```python
from build123d import *

# Parameters (mm, degrees)
MAIN_PROFILE_SKETCH_R    = 1.7
MAIN_EXTRUSION_DEPTH     = 4
DETAIL_EXTRUSION_2_DEPTH = 8


with BuildPart() as part:
    # Main Profile Sketch → Main Extrusion (new body)
    with BuildSketch(Plane.XY.offset(48.5)):
        with BuildLine():
            Line((-110, 55), (-110, -55))
            Line((-110, -55), (-250.126602828, -55))
            ThreePointArc((-250.126602828, -55), (-255, -57.5), (-259.873397172, -55))
            Line((-259.873397172, -55), (-264, -55))
            ThreePointArc((-264, -55), (-275.069801019, -56.026944692), (-275, -44.909830056))
            Line((-275, -44.909830056), (-275, 44.909830056))
            ThreePointArc((-275, 44.909830056), (-275.069801019, 56.026944692), (-264, 55))
            Line((-264, 55), (-259.873397172, 55))
            ThreePointArc((-259.873397172, 55), (-255, 57.5), (-250.126602828, 55))
            Line((-250.126602828, 55), (-110, 55))
        make_face()
        with Locations((-270, -50.5)):
            Circle(MAIN_PROFILE_SKETCH_R, mode=Mode.SUBTRACT)
        with Locations((-255, -51.5)):
            Circle(MAIN_PROFILE_SKETCH_R, mode=Mode.SUBTRACT)
        with Locations((-234, -51)):
            Circle(MAIN_PROFILE_SKETCH_R, mode=Mode.SUBTRACT)
        with Locations((-263, -26.5)):
            Circle(MAIN_PROFILE_SKETCH_R, mode=Mode.SUBTRACT)
        with Locations((-172, -51)):
            Circle(MAIN_PROFILE_SKETCH_R, mode=Mode.SUBTRACT)
        with Locations((-155, -45)):
            Circle(MAIN_PROFILE_SKETCH_R, mode=Mode.SUBTRACT)
        with Locations((-125, -36.5)):
            Circle(MAIN_PROFILE_SKETCH_R, mode=Mode.SUBTRACT)
        with Locations((-167, -26.5)):
            Circle(MAIN_PROFILE_SKETCH_R, mode=Mode.SUBTRACT)
        with Locations((-151.5, -27)):
            Circle(MAIN_PROFILE_SKETCH_R, mode=Mode.SUBTRACT)
        with Locations((-133.5, -27)):
            Circle(MAIN_PROFILE_SKETCH_R, mode=Mode.SUBTRACT)
        with Locations((-116.5, -27)):
            Circle(MAIN_PROFILE_SKETCH_R, mode=Mode.SUBTRACT)
        with Locations((-263, 26.5)):
            Circle(MAIN_PROFILE_SKETCH_R, mode=Mode.SUBTRACT)
        with Locations((-270, 50.5)):
            Circle(MAIN_PROFILE_SKETCH_R, mode=Mode.SUBTRACT)
        with Locations((-255, 51.5)):
            Circle(MAIN_PROFILE_SKETCH_R, mode=Mode.SUBTRACT)
        with Locations((-234, 51)):
            Circle(MAIN_PROFILE_SKETCH_R, mode=Mode.SUBTRACT)
        with Locations((-167, 26.5)):
            Circle(MAIN_PROFILE_SKETCH_R, mode=Mode.SUBTRACT)
        with Locations((-151.5, 27)):
            Circle(MAIN_PROFILE_SKETCH_R, mode=Mode.SUBTRACT)
        with Locations((-133.5, 27)):
            Circle(MAIN_PROFILE_SKETCH_R, mode=Mode.SUBTRACT)
        with Locations((-116.5, 27)):
            Circle(MAIN_PROFILE_SKETCH_R, mode=Mode.SUBTRACT)
        with Locations((-155, 45)):
            Circle(MAIN_PROFILE_SKETCH_R, mode=Mode.SUBTRACT)
        with Locations((-172, 51)):
            Circle(MAIN_PROFILE_SKETCH_R, mode=Mode.SUBTRACT)
        with Locations((-148, 34.5)):
            Circle(MAIN_PROFILE_SKETCH_R, mode=Mode.SUBTRACT)
        with Locations((-125, 36.5)):
            Circle(MAIN_PROFILE_SKETCH_R, mode=Mode.SUBTRACT)
        with Locations((-148, 51.5)):
            Circle(MAIN_PROFILE_SKETCH_R, mode=Mode.SUBTRACT)
    extrude(amount=-MAIN_EXTRUSION_DEPTH)

    # Detail Profile 2 Sketch → Detail Extrusion 2 (add)
    with BuildSketch(Plane.XY.offset(44.5)):
        with BuildLine():
            Line((-265.417424305, -48.5), (-256.374772708, -48.5))
            ThreePointArc((-256.374772708, -48.5), (-257.777296342, -49.717691096), (-258.3, -51.5))
            Line((-258.3, -51.5), (-265.101020514, -51.5))
            ThreePointArc((-265.101020514, -51.5), (-265.027578843, -49.975569032), (-265.417424305, -48.5))
        make_face()
        with BuildLine():
            Line((-253.625227292, -48.5), (-250, -48.5))
            Line((-250, -48.5), (-250, -51.5))
            Line((-250, -51.5), (-251.7, -51.5))
            ThreePointArc((-251.7, -51.5), (-252.222703658, -49.717691096), (-253.625227292, -48.5))
        make_face()
        with BuildLine():
            Line((-227, -51.5), (-175.666060556, -51.5))
            ThreePointArc((-175.666060556, -51.5), (-175.531266062, -49.895391471), (-174.727636339, -48.5))
            Line((-174.727636339, -48.5), (-227, -48.5))
            Line((-227, -48.5), (-227, -51.5))
        make_face()
        with BuildLine():
            Line((-141.5, -48.5), (-141.5, -51.5))
            Line((-141.5, -51.5), (-168.333939444, -51.5))
            ThreePointArc((-168.333939444, -51.5), (-168.468733938, -49.895391471), (-169.272363661, -48.5))
            Line((-169.272363661, -48.5), (-141.5, -48.5))
        make_face()
        with BuildLine():
            Line((-265.101020514, 51.5), (-258.3, 51.5))
            ThreePointArc((-258.3, 51.5), (-257.777296342, 49.717691096), (-256.374772708, 48.5))
            Line((-256.374772708, 48.5), (-265.417424305, 48.5))
            ThreePointArc((-265.417424305, 48.5), (-265.027578843, 49.975569032), (-265.101020514, 51.5))
        make_face()
        with BuildLine():
            Line((-251.7, 51.5), (-250, 51.5))
            Line((-250, 51.5), (-250, 48.5))
            Line((-250, 48.5), (-253.625227292, 48.5))
            ThreePointArc((-253.625227292, 48.5), (-252.222703658, 49.717691096), (-251.7, 51.5))
        make_face()
        with BuildLine():
            Line((-227, 48.5), (-174.727636339, 48.5))
            ThreePointArc((-174.727636339, 48.5), (-175.531266062, 49.895391471), (-175.666060556, 51.5))
            Line((-175.666060556, 51.5), (-227, 51.5))
            Line((-227, 51.5), (-227, 48.5))
        make_face()
        with BuildLine():
            Line((-169.272363661, 48.5), (-150.165640783, 48.5))
            ThreePointArc((-150.165640783, 48.5), (-151.294151704, 49.81519599), (-151.7, 51.5))
            Line((-151.7, 51.5), (-168.333939444, 51.5))
            ThreePointArc((-168.333939444, 51.5), (-168.468733938, 49.895391471), (-169.272363661, 48.5))
        make_face()
        with BuildLine():
            Line((-141.5, 51.5), (-141.5, 48.5))
            Line((-141.5, 48.5), (-145.834359217, 48.5))
            ThreePointArc((-145.834359217, 48.5), (-144.705848296, 49.81519599), (-144.3, 51.5))
            Line((-144.3, 51.5), (-141.5, 51.5))
        make_face()
    extrude(amount=-DETAIL_EXTRUSION_2_DEPTH)


solid = part.part
```
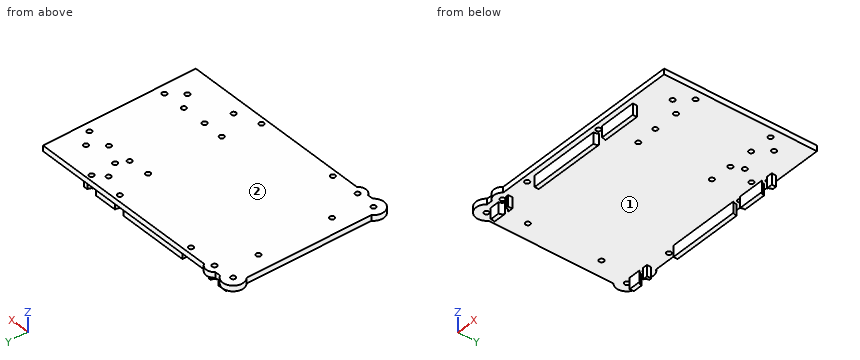
Source: CAD feature listing. Evaluate the final solid. Frame: model axes, mm. Face numbers are marked on the shaded views. Round coordinates to 2 decimals unless told otherwise and drop trailing zeros. Loops run counter-clockwise (first coordinate to the right, second up) from the corner with the lowest first, then second, coordinate; pieces in that order, holes last.
1. Section query D-D on x = -240. Output: boundary loops of the cut face in (y, z), and give its area (3 significant figures).
2. Mould query, pull axis Y, two halves, no side actions, for the marked faces 1 and 2. Classes: released by +Y, released by -Y, zero draft, split by the parting line, or undercut.
3. Section query C-C on y = 12. Output: boundary loops of the cut face in (x, z).
4. Contact query for flat-ended pins moving along their axis: pin 1 (4 mm diameter, centred on x = -151.5, y = -27, fed in from -Z); pin 2 (4.5 mm diameter, centred on y = -14.5, z = 46, fed in from -X); pin 3 (1.4 mm diameter, centred on x = -143, z = 39, fed in from +Y); pin 4 (4.5 mm diameter, centred on x = -116.5, y = -27, fed in from +Z). Output: stop coordinate, or through.
5. Section query B-B on z = 40. Give the number of separate pieces and of enclosed holes in the cut face, and give its area (3 significant figures).
6. Section query A-A on x = -133.5. Output: boundary loops of the cut face in (y, z), and give its area (3 significant figures).
7. Ray query, L1, parallel to Y at x = -234, z = 47.75; L2, parallel to Y at x = -151.5, z = 46.75; L3, parallel to Y at x = -185.5, z = 39.5. Return the intervals inside material, ascending.
Answers below:
1. outline: (-55, 44.5) - (55, 44.5) - (55, 48.5) - (-55, 48.5) - close
1. area: 440 mm2
2. face 1: undercut
2. face 2: zero draft
3. outline: (-275, 44.5) - (-110, 44.5) - (-110, 48.5) - (-275, 48.5) - close
4. pin 1: stops at z = 44.5
4. pin 2: stops at x = -275
4. pin 3: stops at y = 51.5
4. pin 4: stops at z = 48.5
5. separate pieces: 9
5. enclosed holes: 0
5. area: 510 mm2
6. outline: (-55, 44.5) - (-28.7, 44.5) - (-28.7, 48.5) - (-55, 48.5) - close; (-25.3, 44.5) - (25.3, 44.5) - (25.3, 48.5) - (-25.3, 48.5) - close; (28.7, 44.5) - (55, 44.5) - (55, 48.5) - (28.7, 48.5) - close
6. area: 413 mm2
7. L1: y = -55 to -52.7, -49.3 to 49.3, 52.7 to 55
7. L2: y = -55 to -28.7, -25.3 to 25.3, 28.7 to 55
7. L3: y = -51.5 to -48.5, 48.5 to 51.5
